For this review, take the finished solid that the model builds, in its own axes (mm). A direction names the side the tool comes from. Coordinates: 2 decimals unless noted, no trailing zeros. Loops run counter-clockwise (first coordinate to the right, second up) from the corner with the lowest first, then second, coordinate; pieces in that order, holes last. Notation, with made-up numbers: (78, 49.25) -> (98, 49.25) arc R18 ccw to (98, 61.25) -> close; hole circle Ø10 at (-7, -30.75). An arc over 180 degrees is marked (long way). One line per item, written item: value.
from build123d import *

# Parameters (mm, degrees)
SKETCH2_R                = 60
BOSS_EXTRUDE1_DEPTH      = 15
BOSS_EXTRUDE1_DEPTH_BACK = 15
SKETCH3_R                = 40
CUT_EXTRUDE1_DEPTH       = 11.5
SKETCH4_R                = 21
BOSS_EXTRUDE2_DEPTH      = 6
SKETCH5_R                = 7.5
CUT_EXTRUDE2_DEPTH       = 20


with BuildPart() as part:
    # Sketch2 → Boss-Extrude1 (new body, two sides)
    with BuildSketch(Plane(origin=(0, 0, 0), x_dir=(1, 0, 0), z_dir=(0, 1, 0))) as boss_extrude1_sk:
        Circle(SKETCH2_R)
    extrude(amount=BOSS_EXTRUDE1_DEPTH)
    extrude(boss_extrude1_sk.sketch, amount=-BOSS_EXTRUDE1_DEPTH_BACK)

    # Sketch3 → Cut-Extrude1 (cut)
    with BuildSketch(Plane(origin=(0, 15, 0), x_dir=(1, 0, 0), z_dir=(0, 1, 0))):
        Circle(SKETCH3_R)
    cut_extrude1 = extrude(amount=-CUT_EXTRUDE1_DEPTH, mode=Mode.SUBTRACT)

    # Sketch4 → Boss-Extrude2 (add)
    with BuildSketch(Plane(origin=(0, 3.5, 0), x_dir=(1, 0, 0), z_dir=(0, 1, 0))):
        Circle(SKETCH4_R)
    boss_extrude2 = extrude(amount=BOSS_EXTRUDE2_DEPTH)

    # Sketch5 → Cut-Extrude2 (cut)
    with BuildSketch(Plane(origin=(0, 9.5, 0), x_dir=(1, 0, 0), z_dir=(0, 1, 0))):
        Circle(SKETCH5_R)
    cut_extrude2 = extrude(amount=-CUT_EXTRUDE2_DEPTH, mode=Mode.SUBTRACT)

    # Mirror1: Cut-Extrude1, Boss-Extrude2, Cut-Extrude2 across plane
    add(cut_extrude1.mirror(Plane.ZX), mode=Mode.SUBTRACT)
    add(boss_extrude2.mirror(Plane.ZX))
    add(cut_extrude2.mirror(Plane.ZX), mode=Mode.SUBTRACT)


solid = part.part
1. The part is to be moulded in two halves that separate along Z. For faces 1 (the cylindrical face through (-59.94, 0.21, -2.64)), 2 (the cylindrical face through (-8.67, -9.33, 39.05)), 3 (the flat face through (12, -15, 39)), say which applies: pulls with the +Z half, pulls with the -Z half, needs draft (parallel to the pull), parting line crosses it, or undercut.
Return value:
face 1: parting line crosses it
face 2: undercut
face 3: needs draft
2. Take a section at A-A, the plane z = 0. Give the boundary of the cut face in (x, y).
Return value:
outline: (-60, -15) -> (-40, -15) -> (-40, -3.5) -> (-21, -3.5) -> (-21, -9.5) -> (-7.5, -9.5) -> (-7.5, 9.5) -> (-21, 9.5) -> (-21, 3.5) -> (-40, 3.5) -> (-40, 15) -> (-60, 15) -> close; (7.5, -9.5) -> (21, -9.5) -> (21, -3.5) -> (40, -3.5) -> (40, -15) -> (60, -15) -> (60, 15) -> (40, 15) -> (40, 3.5) -> (21, 3.5) -> (21, 9.5) -> (7.5, 9.5) -> close
3. For faces 4 (the cylindrical face through (-7.493, -0.133, -0.33)), 5 (the cylindrical face through (20.03, -6.46, -6.31)), 6 (the cylindrical face through (20.03, 6.46, -6.31)), list the 3-axis set-ups (+Z, -Z, +X, -X, +Y, -Y) from which the entire face can be reached by the end or side of a thin tool; tool diameter is ignored.
Return value:
face 4: +Y, -Y
face 5: -Y
face 6: +Y
4. Take a section at C-C, the plane y = 7.75. Give the boundary of the cut face in (x, z), and give its area (3 significant figures).
Return value:
outline: circle Ø120 at (0, 0); circle Ø42 at (0, 0); hole circle Ø80 at (0, 0); hole circle Ø15 at (0, 0)
area: 7,490 mm2
5. Take a section at B-B, the plane x = 0. Give the boundary of the cut face in (y, z), and give its area (3 significant figures).
Return value:
outline: (-15, -60) -> (15, -60) -> (15, -40) -> (3.5, -40) -> (3.5, -21) -> (9.5, -21) -> (9.5, -7.5) -> (-9.5, -7.5) -> (-9.5, -21) -> (-3.5, -21) -> (-3.5, -40) -> (-15, -40) -> close; (-15, 40) -> (-3.5, 40) -> (-3.5, 21) -> (-9.5, 21) -> (-9.5, 7.5) -> (9.5, 7.5) -> (9.5, 21) -> (3.5, 21) -> (3.5, 40) -> (15, 40) -> (15, 60) -> (-15, 60) -> close
area: 1,980 mm2
6. Insertion check: pin 1 Ø12 at (y, z) = (-7, -12) entering from -X; pin 2 Ø4 at (x, y) = (-9, -7) entering from -Z; pin 3 Ø21 at (x, z) = (8, -4) entering from +Y. Each pin has a flat end and moves straight along its axis. Give the tip position at first contact, or say it passes through.
Return value:
pin 1: stops at x = -59.7
pin 2: stops at z = -59.59
pin 3: stops at y = 9.5
7. Take a section at D-D, the plane x = -13. Give the boundary of the cut face in (y, z), and give its area (3 significant figures).
Return value:
outline: (-15, -58.57) -> (15, -58.57) -> (15, -37.83) -> (3.5, -37.83) -> (3.5, -16.49) -> (9.5, -16.49) -> (9.5, 16.49) -> (3.5, 16.49) -> (3.5, 37.83) -> (15, 37.83) -> (15, 58.57) -> (-15, 58.57) -> (-15, 37.83) -> (-3.5, 37.83) -> (-3.5, 16.49) -> (-9.5, 16.49) -> (-9.5, -16.49) -> (-3.5, -16.49) -> (-3.5, -37.83) -> (-15, -37.83) -> close
area: 2,170 mm2
8. To check wall thickness, follow probe 1 along X at (y, z) = (7.5, 0); probe 2 along Z at (x, y) = (0, 0.5); probe 3 along X at (y, z) = (11.25, 0). State the ranges of each line that lie inside material, in increasing order. Write a range as from..to.
Return value:
probe 1: x = -60..-40, -21..-7.5, 7.5..21, 40..60
probe 2: z = -60..-7.5, 7.5..60
probe 3: x = -60..-40, 40..60
